Check sheet for the modelled part. Datum: model origin and axes. Units: mm. A direction names the side the tool comes from. Round coordinates to 2 decimals unless told otherwise and drop trailing zeros. Order: outer loops, then holes, each group sorted by start corner. A loop starts at its lowest first (then second) coordinate and runs counter-clockwise, first axis right, second up. Notation, with made-up numbers: (47.5, 43) -> (78.5, 43) arc R20 ccw to (78.5, 50) -> close; hole circle Ø10 at (1, 69.25). An arc over 180 degrees is marked (long way). Answer in a Markdown table with one row per item.
```python
from build123d import *

# Parameters (mm, degrees)
EXTRU_MINCE1_DEPTH           = 2.3
CONG_1_R                     = 2.3
ESQUISSE2_W                  = 120
ESQUISSE2_H                  = 49.6
BOSS_EXTRU_1_DEPTH           = 2.3
R_P_TITION_START             = 117.7
R_P_TITION_LIN_AIRE1_DEPTH   = 4.6
R_P_TITION_START_2           = 37.7
R_P_TITION_LIN_AIRE1_2_DEPTH = 4.6
R_P_TITION_START_3           = 77.7
R_P_TITION_LIN_AIRE1_3_DEPTH = 4.6
CONG_2_R                     = 2.3
BOSS_EXTRU_2_START           = -30
BOSS_EXTRU_2_OUTLINE_R       = 5
BOSS_EXTRU_2_OUTLINE_R_2     = 3.75
BOSS_EXTRU_2_OUTLINE_R_3     = 3
BOSS_EXTRU_2_DEPTH           = 10


# Read off the part's stored shape, not the designer's step: Répétition linéaire1, Boss.-Extru.2
with BuildPart() as part:
    # Esquisse1 → Extru.-Mince1 (new, symmetric)
    with BuildSketch(Plane.XY):
        Polygon((-4.3, -57), (-4.3, -47.3), (2.3, -47.3), (2.3, 2.3), (-8.9, 2.3), (-8.9, -12), (-4.3, -12), (-4.3, -2.3), (-2.3, -2.3), (-2.3, -42.7), (-8.9, -42.7), (-8.9, -57), align=None)
    extrude(amount=EXTRU_MINCE1_DEPTH, both=True)

    # Congé1
    cong_1_edges = [part.edges().sort_by_distance(p)[0] for p in [
        (-6.6, -57, -2.3),
        (-4.3, -52.15, -2.3),
        (-1, -47.3, -2.3),
        (2.3, -22.5, -2.3),
        (-3.3, 2.3, -2.3),
        (-8.9, -4.85, -2.3),
        (-6.6, -12, -2.3),
        (-4.3, -7.15, -2.3),
        (-3.3, -2.3, -2.3),
        (-2.3, -22.5, -2.3),
        (-5.6, -42.7, -2.3),
        (-8.9, -49.85, -2.3),
        (-5.6, -42.7, 2.3),
        (-2.3, -22.5, 2.3),
        (-3.3, -2.3, 2.3),
        (-4.3, -7.15, 2.3),
        (-6.6, -12, 2.3),
        (-8.9, -4.85, 2.3),
        (-3.3, 2.3, 2.3),
        (2.3, -22.5, 2.3),
        (-1, -47.3, 2.3),
        (-4.3, -52.15, 2.3),
        (-6.6, -57, 2.3),
        (-8.9, -49.85, 2.3),
    ]]
    fillet(cong_1_edges, radius=CONG_1_R - 0.0001)  # a hair under: the kernel refuses the full size

    # Esquisse2 → Boss.-Extru.1 (add)
    with BuildSketch(Plane(origin=(0, 0, 0), x_dir=(0, 0, -1), z_dir=(1, 0, 0))):
        with Locations((-60, -22.5)):
            Rectangle(ESQUISSE2_W, ESQUISSE2_H)
    extrude(amount=BOSS_EXTRU_1_DEPTH)

    # Répétition linéaire1 outline → Répétition linéaire1 (add)
    with BuildSketch(Plane.XY.offset(R_P_TITION_START)):
        Polygon((-8.9, 2.3), (-8.9, -12), (-4.3, -12), (-4.3, -2.3), (-2.3, -2.3), (-2.3, -42.7), (-8.9, -42.7), (-8.9, -57), (-4.3, -57), (-4.3, -47.3), (2.3, -47.3), (2.3, 2.3), align=None)
    extrude(amount=R_P_TITION_LIN_AIRE1_DEPTH)

    # R_p_tition lin_aire1 2 outline → R_p_tition lin_aire1 2 (add)
    with BuildSketch(Plane.XY.offset(R_P_TITION_START_2)):
        Polygon((0, 2.3), (-8.9, 2.3), (-8.9, -12), (-4.3, -12), (-4.3, -2.3), (-2.3, -2.3), (-2.3, -42.7), (-8.9, -42.7), (-8.9, -57), (-4.3, -57), (-4.3, -47.3), (0, -47.3), align=None)
    extrude(amount=R_P_TITION_LIN_AIRE1_2_DEPTH)

    # R_p_tition lin_aire1 3 outline → R_p_tition lin_aire1 3 (add)
    with BuildSketch(Plane.XY.offset(R_P_TITION_START_3)):
        Polygon((0, 2.3), (-8.9, 2.3), (-8.9, -12), (-4.3, -12), (-4.3, -2.3), (-2.3, -2.3), (-2.3, -42.7), (-8.9, -42.7), (-8.9, -57), (-4.3, -57), (-4.3, -47.3), (0, -47.3), align=None)
    extrude(amount=R_P_TITION_LIN_AIRE1_3_DEPTH)

    # Congé2
    cong_2_edges = [part.edges().sort_by_distance(p)[0] for p in [
        (-2.15, -47.3, 82.3),
        (-4.45, 2.3, 82.3),
        (-4.3, -7.15, 82.3),
        (-3.3, -2.3, 82.3),
        (-2.3, -22.5, 82.3),
        (-5.6, -42.7, 82.3),
        (-8.9, -49.85, 82.3),
        (-4.45, 2.3, 77.7),
        (-2.15, -47.3, 77.7),
        (-4.3, -52.15, 77.7),
        (-6.6, -57, 77.7),
        (-6.6, -12, 77.7),
        (-8.9, -4.85, 77.7),
        (-8.9, -49.85, 77.7),
        (-6.6, -57, 82.3),
        (-4.3, -52.15, 82.3),
        (-8.9, -4.85, 82.3),
        (-6.6, -12, 82.3),
        (-4.3, -7.15, 77.7),
        (-3.3, -2.3, 77.7),
        (-2.3, -22.5, 77.7),
        (-5.6, -42.7, 77.7),
        (2.3, -22.5, 122.3),
        (-1, -47.3, 122.3),
        (-3.3, 2.3, 122.3),
        (-4.45, 2.3, 117.7),
        (-2.15, -47.3, 117.7),
        (-4.3, -52.15, 117.7),
        (-6.6, -57, 117.7),
        (-6.6, -12, 117.7),
        (-8.9, -4.85, 117.7),
        (-8.9, -49.85, 117.7),
        (-6.6, -57, 122.3),
        (-4.3, -52.15, 122.3),
        (-8.9, -4.85, 122.3),
        (-6.6, -12, 122.3),
        (-4.3, -7.15, 117.7),
        (-3.3, -2.3, 117.7),
        (-2.3, -22.5, 117.7),
        (-5.6, -42.7, 117.7),
        (-8.9, -49.85, 122.3),
        (-4.3, -7.15, 122.3),
        (-3.3, -2.3, 122.3),
        (-2.3, -22.5, 122.3),
        (-5.6, -42.7, 122.3),
        (-2.15, -47.3, 42.3),
        (-4.45, 2.3, 42.3),
        (-4.3, -7.15, 42.3),
        (-3.3, -2.3, 42.3),
        (-2.3, -22.5, 42.3),
        (-5.6, -42.7, 42.3),
        (-8.9, -49.85, 42.3),
        (-4.45, 2.3, 37.7),
        (-2.15, -47.3, 37.7),
        (-4.3, -52.15, 37.7),
        (-6.6, -57, 37.7),
        (-6.6, -12, 37.7),
        (-8.9, -4.85, 37.7),
        (-8.9, -49.85, 37.7),
        (-6.6, -57, 42.3),
        (-4.3, -52.15, 42.3),
        (-8.9, -4.85, 42.3),
        (-6.6, -12, 42.3),
        (-4.3, -7.15, 37.7),
        (-3.3, -2.3, 37.7),
        (-2.3, -22.5, 37.7),
        (-5.6, -42.7, 37.7),
    ]]
    fillet(cong_2_edges, radius=CONG_2_R - 0.0001)  # a hair under: the kernel refuses the full size

    # Boss.-Extru.2 outline → Boss.-Extru.2 (add)
    with BuildSketch(Plane(origin=(0, 0, 0), x_dir=(1, 0, 0), z_dir=(0, 1, 0)).offset(BOSS_EXTRU_2_START)):
        with BuildLine():
            Line((2.3, -120), (22.3, -120))
            ThreePointArc((22.3, -120), (29.371067812, -117.071067812), (32.3, -110))
            Line((32.3, -110), (32.3, -90))
            ThreePointArc((32.3, -90), (30.71604952, -84.599063926), (26.465977905, -80.909090909))
            ThreePointArc((26.465977905, -80.909090909), (25.882575695, -80), (26.465977905, -79.090909091))
            ThreePointArc((26.465977905, -79.090909091), (30.71604952, -75.400936074), (32.3, -70))
            Line((32.3, -70), (32.3, -50))
            ThreePointArc((32.3, -50), (30.71604952, -44.599063926), (26.465977905, -40.909090909))
            ThreePointArc((26.465977905, -40.909090909), (25.882575695, -40), (26.465977905, -39.090909091))
            ThreePointArc((26.465977905, -39.090909091), (30.71604952, -35.400936074), (32.3, -30))
            Line((32.3, -30), (32.3, -10))
            ThreePointArc((32.3, -10), (29.371067812, -2.928932188), (22.3, 0))
            Line((22.3, 0), (2.3, 0))
            Line((2.3, 0), (2.3, -120))
        make_face()
        with Locations((17.3, -100)):
            Circle(BOSS_EXTRU_2_OUTLINE_R, mode=Mode.SUBTRACT)
        with Locations((17.3, -60)):
            Circle(BOSS_EXTRU_2_OUTLINE_R_2, mode=Mode.SUBTRACT)
        with Locations((17.3, -20)):
            Circle(BOSS_EXTRU_2_OUTLINE_R_3, mode=Mode.SUBTRACT)
    extrude(amount=BOSS_EXTRU_2_DEPTH)


solid = part.part
```
(1) Section check A-A on z = 100. Record the boundary of the cut face in (x, y), plus the area to 3 significant figures.
Solutions:
| item | result |
|---|---|
| outline | (0, -47.3) -> (2.3, -47.3) -> (2.3, -30) -> (12.3, -30) -> (12.3, -20) -> (2.3, -20) -> (2.3, 2.3) -> (0, 2.3) -> close; (22.3, -30) -> (32.3, -30) -> (32.3, -20) -> (22.3, -20) -> close |
| area | 314 mm^2 |
(2) Tool access check on faces 1 (the cylindrical face through (-6.57, -56.57, 78.66)), 2 (the cylindrical face through (-4.99, -50.92, 81.64)), 3 (the cylindrical face through (-3.254, -1.298, 121.898)), 4 (the cylindrical face through (-1.61, -22.81, 78.36)). Record the directions out of +Z, -Z, +X, -X, +Y, -Y that give a thin tool (end or side, any length) a straight path to the whole face; none if there is none.
Solutions:
| item | result |
|---|---|
| face 1 | +X, -X, -Y |
| face 2 | -Y |
| face 3 | +Z |
| face 4 | none |
(3) Draft check along Z on faces 5 (the cylindrical face through (-6.57, -11.57, 41.34)), 6 (the cylindrical face through (1.61, -22.15, 121.64)), 7 (the flat face through (32.3, -25, 100)), 8 (the cylindrical face through (-6.57, -56.57, 81.34)). Enter one of: pulls with the +Z half, pulls with the -Z half, needs draft (parallel to the pull), parting line crosses it, or undercut.
Solutions:
| item | result |
|---|---|
| face 5 | undercut |
| face 6 | pulls with the +Z half |
| face 7 | needs draft |
| face 8 | undercut |
(4) Section check B-B on y = -50. Give the number of separate pieces and of enclosed holes in the cut face, plus the area to 3 significant figures.
Solutions:
| item | result |
|---|---|
| separate pieces | 4 |
| enclosed holes | 0 |
| area | 66.5 mm^2 |
(5) Depth check by flat-ended pin: pin 1 Ø12 at (y, z) = (-13.5, 72) entering from +X; pin 2 Ø8 at (x, y) = (15, -27) entering from -Z; pin 3 Ø10 at (x, z) = (17.3, 60) entering from -Y. Enter the tip coordinate at first touch or a pass-through.
Solutions:
| item | result |
|---|---|
| pin 1 | x = 2.3 |
| pin 2 | z = 0 |
| pin 3 | y = -30 |
(6) Section check C-C on x = 17.3. Record the boundary of the cut face in (y, z).
Solutions:
| item | result |
|---|---|
| outline | (-30, 0) -> (-20, 0) -> (-20, 17) -> (-30, 17) -> close; (-30, 23) -> (-20, 23) -> (-20, 56.25) -> (-30, 56.25) -> close; (-30, 63.75) -> (-20, 63.75) -> (-20, 95) -> (-30, 95) -> close; (-30, 105) -> (-20, 105) -> (-20, 120) -> (-30, 120) -> close |
(7) Scan lines: probe 1 along Z at (x, y) = (17, -24); probe 2 along X at (y, z) = (-25.75, 60); probe 3 along X at (y, z) = (-23, 20). Record each from-to range of solid material in increasing order. Write a range as from..to.
Solutions:
| item | result |
|---|---|
| probe 1 | 0..17.02, 22.98..56.26, 63.74..95.01, 104.99..120 |
| probe 2 | 0..13.55, 21.05..32.3 |
| probe 3 | 0..14.3, 20.3..32.3 |
